Here's how the part is built. I have some questions about the finished solid (model axes, mm). A direction names the side the tool comes from. Coordinates: 2 decimals unless noted, no trailing zeros. Write each loop counter-clockwise with the first axis right and the second up, starting at its lowest first coordinate (ties: lowest second). Pieces come first, ordered by that corner, then holes. Notation, with made-up numbers: (11.5, 60) -> (24.5, 60) arc R13 cw to (24.5, 66) -> close; hole circle Ø8 at (7, 12). An arc over 180 degrees is marked (long way). Put each result on its own line as item: value.
```python
from build123d import *

# Parameters (mm, degrees)
SKETCH1_W           = 76.2
SKETCH1_H           = 25.4
SKETCH1_W_2         = 69.85
SKETCH1_H_2         = 19.05
EXTRUDE_THIN1_DEPTH = 50.8
SKETCH2_R           = 24.97201
CUT_EXTRUDE1_DEPTH  = 52.578
CUT_EXTRUDE2_DEPTH  = 26.4
SKETCH6_R           = 3.175
CUT_EXTRUDE3_DEPTH  = 77.2
SKETCH7_R           = 3.175
CUT_EXTRUDE4_DEPTH  = 77.2


with BuildPart() as part:
    # Sketch1 → Extrude-Thin1 (new body, symmetric)
    with BuildSketch(Plane(origin=(0, 0, 0), x_dir=(1, 0, 0), z_dir=(0, 1, 0))):
        with Locations((38.1, 12.7)):
            Rectangle(SKETCH1_W, SKETCH1_H)
        with Locations((38.1, 12.7)):
            Rectangle(SKETCH1_W_2, SKETCH1_H_2, mode=Mode.SUBTRACT)
    extrude(amount=EXTRUDE_THIN1_DEPTH, both=True)

    # Sketch2 → Cut-Extrude1 (cut)
    with BuildSketch(Plane(origin=(0, 0, -25.4), x_dir=(-1, 0, 0), z_dir=(0, 0, -1))):
        with Locations((-38.1, -12.7)):
            Circle(SKETCH2_R)
    extrude(amount=-CUT_EXTRUDE1_DEPTH, mode=Mode.SUBTRACT)

    # Sketch5 → Cut-Extrude2 (cut, through all)
    with BuildSketch(Plane(origin=(0, 0, -25.4), x_dir=(-1, 0, 0), z_dir=(0, 0, -1))):
        Polygon((0, 50.8), (-76.2, 50.8), (-76.2, 46.1645), (-63.5, 46.1645), (-12.7, 46.1645), (0, 46.1645), align=None)
        with BuildLine():
            Line((-12.7, 46.1645), (-63.5, 46.1645))
            Line((-63.5, 46.1645), (-63.5, 13.683575837))
            ThreePointArc((-63.5, 13.683575837), (-61.664047105, 10.804760481), (-58.279478519, 11.255311669))
            ThreePointArc((-58.279478519, 11.255311669), (-38.1, 18.62201), (-17.920521481, 11.255311669))
            ThreePointArc((-17.920521481, 11.255311669), (-14.535952895, 10.804760481), (-12.7, 13.683575837))
            Line((-12.7, 13.683575837), (-12.7, 46.1645))
        make_face()
    extrude(amount=-CUT_EXTRUDE2_DEPTH, mode=Mode.SUBTRACT)

    # Sketch6 → Cut-Extrude3 (cut, through all)
    with BuildSketch(Plane.ZY):
        with Locations((-12.7, 31.75)):
            Circle(SKETCH6_R)
    extrude(amount=-CUT_EXTRUDE3_DEPTH, mode=Mode.SUBTRACT)

    # Sketch7 → Cut-Extrude4 (cut, through all)
    with BuildSketch(Plane.ZY):
        with Locations((-12.7, -12.7)):
            Circle(SKETCH7_R)
    extrude(amount=-CUT_EXTRUDE4_DEPTH, mode=Mode.SUBTRACT)


solid = part.part
```
Item 1: For P1, Ø5, axis at x = 40, y = 21, coming from the +Z side; P2, Ø6, axis at x = 57.5, z = -19.5, coming from the +Y side; P3, Ø1, axis at x = 34.5, z = -21, coming from the +Y side, each with a flat end and sliding along its axis, tell me the tip position at first contact or that it passes through.
Output:
P1: stops at z = 0
P2: stops at y = 12.83
P3: passes through
Item 2: Imagine slicing it at C-C on z = -18. Write out the boundary of the cut face in (x, y) (1 decimal), then the cut area to 3 significant figures.
Output:
outline: (0, -50.8) -> (3.2, -50.8) -> (3.2, 46.2) -> (0, 46.2) -> close; (73, -50.8) -> (76.2, -50.8) -> (76.2, 46.2) -> (73, 46.2) -> close
area: 616 mm²
Item 3: If we mould it in two halves opening along X, with no side actions, what happens to faces 1 (the cylindrical face through (14.582, 10.784, -23.835)), 2 (the cylindrical face through (1.6, -15.5, -11.2)), 3 (the flat face through (0, -2, -13))? For each: released by +X, released by -X, zero draft, split by the parting line, or undercut.
Output:
face 1: undercut
face 2: zero draft
face 3: released by -X
Item 4: Which directions (+Z, -Z, +X, -X, +Y, -Y) give clear straight access to the entire face, cutting with the end or side of a thin tool? Please do faces 4 (the flat face through (12.7, 30, -24)), 5 (the flat face through (14, -23, -3.175)), 6 (the flat face through (76.2, -2, -13)).
Output:
face 4: +Z, -Z, +Y
face 5: +Y, -Y
face 6: +Z, -Z, +X, +Y, -Y
Item 5: Imagine slicing it at D-D on y = -41. Write out the boundary of the cut face in (x, z) (3 decimals), then the cut area to 3 significant figures.
Output:
outline: (0, -25.4) -> (76.2, -25.4) -> (76.2, 0) -> (0, 0) -> close; hole (3.175, -22.225) -> (73.025, -22.225) -> (73.025, -3.175) -> (3.175, -3.175) -> close
area: 605 mm²
Item 6: Imagine slicing it at B-B on x = 38.1. Write out the boundary of the cut face in (y, z) (3 decimals), then the cut area to 3 significant figures.
Output:
outline: (-50.8, -25.4) -> (-37.672, -25.4) -> (-37.672, -22.225) -> (-50.8, -22.225) -> close; (-50.8, -3.175) -> (-37.672, -3.175) -> (-37.672, 0) -> (-50.8, 0) -> close; (12.272, -25.4) -> (18.622, -25.4) -> (18.622, -22.225) -> (12.272, -22.225) -> close; (12.272, -3.175) -> (18.622, -3.175) -> (18.622, 0) -> (12.272, 0) -> close
area: 124 mm²
Item 7: Please list where these lines run through material, in increasing order: line 1 along X through (y, z) = (-36, -18) (3 decimals); line 2 along Y through (x, z) = (74.15, -12.7) (1 decimal); line 3 along Z through (x, y) = (11, 30) (3 decimals). Write a range as from..to.
Output:
line 1: x = 0..3.175, 73.025..76.2
line 2: y = -50.8..-15.9, -9.5..28.6, 34.9..46.2
line 3: z = -25.4..-22.225, -3.175..0
Item 8: Imagine slicing it at A-A on y = 24. Write out the boundary of the cut face in (x, z) (3 decimals), then the cut area to 3 significant figures.
Output:
outline: (0, -25.4) -> (12.7, -25.4) -> (12.7, -22.225) -> (3.175, -22.225) -> (3.175, -3.175) -> (12.7, -3.175) -> (12.7, 0) -> (0, 0) -> close; (63.5, -25.4) -> (76.2, -25.4) -> (76.2, 0) -> (63.5, 0) -> (63.5, -3.175) -> (73.025, -3.175) -> (73.025, -22.225) -> (63.5, -22.225) -> close
area: 282 mm²
